CAD build for the part. Positions are in the model's coordinates, mm. Face numbers are marked on the shaded views. A direction names the side the tool comes from. Coordinates: 2 decimals unless noted, no trailing zeros. Order: outer loops, then holes, each group sorted by start corner. A loop starts at its lowest first (then second) coordinate and runs counter-clockwise, first axis right, second up. Notation, with made-up numbers: (-30, 64) - (17, 64) arc R36 cw to (17, 103) - close; hole circle Ø5 at (88, 70.5). An arc over 180 degrees is marked (long way). Use one line per item in the form item = value.
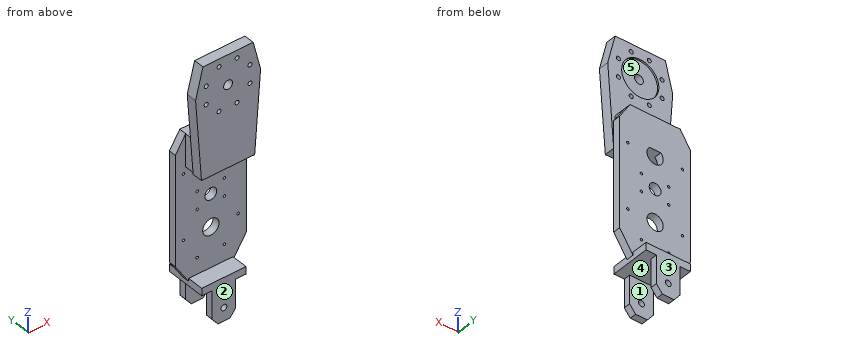
```python
from build123d import *

# Parameters (mm, degrees)
SK_KNEE_PLATE_R         = 2.75
SK_KNEE_PLATE_R_2       = 6
KNEE_PLATE_DEPTH        = 14
SK_KNEE_PILOT_RECESS_R  = 25.15
KNEE_PILOT_RECESS_DEPTH = 2.2
SK_JOGGLE_W             = 68
SK_JOGGLE_H             = 39
JOGGLE_DEPTH            = 44
SK_WEB_R                = 1.7
SK_WEB_R_2              = 11
SK_WEB_R_3              = 8
WEB_DEPTH               = 10
SK_FORK_BAR_W           = 60
SK_FORK_BAR_H           = 54
FORK_BAR_DEPTH          = 10
SK_TINE_LAT_R           = 4
TINE_LAT_DEPTH          = 9
SK_TINE_MED_R           = 4
TINE_MED_DEPTH          = 9


with BuildPart() as part:
    # SK_Knee_Plate → Knee_Plate (new body)
    with BuildSketch(Plane(origin=(0, -34, 0), x_dir=(1, 0, 0), z_dir=(0, 1, 0))):
        Polygon((-34, -40), (34, -40), (44, 0), (36, 110), (-36, 110), (-44, 0), align=None)
        with Locations(Location((29.56414504, 12.245869836, 0), (0, 0, 90))):
            Circle(SK_KNEE_PLATE_R, mode=Mode.SUBTRACT)
        with Locations(Location((12.245869836, 29.56414504, 0), (0, 0, 90))):
            Circle(SK_KNEE_PLATE_R, mode=Mode.SUBTRACT)
        with Locations(Location((-12.245869836, 29.56414504, 0), (0, 0, 90))):
            Circle(SK_KNEE_PLATE_R, mode=Mode.SUBTRACT)
        with Locations(Location((-29.56414504, 12.245869836, 0), (0, 0, 90))):
            Circle(SK_KNEE_PLATE_R, mode=Mode.SUBTRACT)
        with Locations(Location((-29.56414504, -12.245869836, 0), (0, 0, 90))):
            Circle(SK_KNEE_PLATE_R, mode=Mode.SUBTRACT)
        with Locations(Location((-12.245869836, -29.56414504, 0), (0, 0, 90))):
            Circle(SK_KNEE_PLATE_R, mode=Mode.SUBTRACT)
        with Locations(Location((12.245869836, -29.56414504, 0), (0, 0, 90))):
            Circle(SK_KNEE_PLATE_R, mode=Mode.SUBTRACT)
        with Locations(Location((29.56414504, -12.245869836, 0), (0, 0, 90))):
            Circle(SK_KNEE_PLATE_R, mode=Mode.SUBTRACT)
        with Locations(Location((0, 0, 0), (0, 0, 90))):
            Circle(SK_KNEE_PLATE_R_2, mode=Mode.SUBTRACT)
    extrude(amount=KNEE_PLATE_DEPTH)

    # SK_Knee_Pilot_Recess → Knee_Pilot_Recess (cut)
    with BuildSketch(Plane(origin=(0, -20, 0), x_dir=(1, 0, 0), z_dir=(0, 1, 0))):
        with Locations(Location((0, 0, 0), (0, 0, 270))):
            Circle(SK_KNEE_PILOT_RECESS_R)
    extrude(amount=-KNEE_PILOT_RECESS_DEPTH, mode=Mode.SUBTRACT)

    # SK_Joggle → Joggle (add)
    with BuildSketch(Plane.XY.offset(-110)):
        with Locations((0, -14.5)):
            Rectangle(SK_JOGGLE_W, SK_JOGGLE_H)
    extrude(amount=JOGGLE_DEPTH)

    # SK_Web → Web (add)
    with BuildSketch(Plane(origin=(0, -5, 0), x_dir=(1, 0, 0), z_dir=(0, 1, 0))):
        Polygon((-34, 66), (34, 66), (48, 88), (48, 236), (30, 264), (-30, 264), (-48, 236), (-48, 88), align=None)
        with Locations(Location((37, 118, 0), (0, 0, 270))):
            Circle(SK_WEB_R, mode=Mode.SUBTRACT)
        with Locations(Location((18.5, 150.04293994, 0), (0, 0, 270))):
            Circle(SK_WEB_R, mode=Mode.SUBTRACT)
        with Locations(Location((-18.5, 150.04293994, 0), (0, 0, 270))):
            Circle(SK_WEB_R, mode=Mode.SUBTRACT)
        with Locations(Location((-37, 118, 0), (0, 0, 270))):
            Circle(SK_WEB_R, mode=Mode.SUBTRACT)
        with Locations((-18.5, 85.95706006)):
            Circle(SK_WEB_R, mode=Mode.SUBTRACT)
        with Locations((18.5, 85.95706006)):
            Circle(SK_WEB_R, mode=Mode.SUBTRACT)
        with Locations(Location((37, 206, 0), (0, 0, 270))):
            Circle(SK_WEB_R, mode=Mode.SUBTRACT)
        with Locations(Location((18.5, 238.04293994, 0), (0, 0, 270))):
            Circle(SK_WEB_R, mode=Mode.SUBTRACT)
        with Locations(Location((-18.5, 238.04293994, 0), (0, 0, 270))):
            Circle(SK_WEB_R, mode=Mode.SUBTRACT)
        with Locations(Location((-37, 206, 0), (0, 0, 270))):
            Circle(SK_WEB_R, mode=Mode.SUBTRACT)
        with Locations(Location((-18.5, 173.95706006, 0), (0, 0, 270))):
            Circle(SK_WEB_R, mode=Mode.SUBTRACT)
        with Locations(Location((18.5, 173.95706006, 0), (0, 0, 270))):
            Circle(SK_WEB_R, mode=Mode.SUBTRACT)
        with Locations((0, 118)):
            Circle(SK_WEB_R_2, mode=Mode.SUBTRACT)
        with Locations(Location((0, 206, 0), (0, 0, 270))):
            Circle(SK_WEB_R_2, mode=Mode.SUBTRACT)
        with Locations(Location((0, 162, 0), (0, 0, 270))):
            Circle(SK_WEB_R_3, mode=Mode.SUBTRACT)
    extrude(amount=WEB_DEPTH)

    # SK_Fork_Bar → Fork_Bar (add)
    with BuildSketch(Plane.XY.offset(-270)):
        Rectangle(SK_FORK_BAR_W, SK_FORK_BAR_H)
    extrude(amount=FORK_BAR_DEPTH)

    # SK_Tine_Lat → Tine_Lat (add)
    with BuildSketch(Plane(origin=(0, 18, 0), x_dir=(1, 0, 0), z_dir=(0, 1, 0))):
        Polygon((-16, 260), (16, 260), (16, 308), (8, 318), (-8, 318), (-16, 308), align=None)
        with Locations(Location((0, 300, 0), (0, 0, 270))):
            Circle(SK_TINE_LAT_R, mode=Mode.SUBTRACT)
    extrude(amount=TINE_LAT_DEPTH)

    # SK_Tine_Med → Tine_Med (add)
    with BuildSketch(Plane(origin=(0, -27, 0), x_dir=(1, 0, 0), z_dir=(0, 1, 0))):
        Polygon((-16, 260), (16, 260), (16, 308), (8, 318), (-8, 318), (-16, 308), align=None)
        with Locations(Location((0, 300, 0), (0, 0, 270))):
            Circle(SK_TINE_MED_R, mode=Mode.SUBTRACT)
    extrude(amount=TINE_MED_DEPTH)


solid = part.part
```
Item 1: Cut at B-B, the plane z = -291. Write the cut outline in (x, y), plus the area to 3 significant figures.
Derived:
outline = (-16, -27) - (16, -27) - (16, -18) - (-16, -18) - close; (-16, 18) - (16, 18) - (16, 27) - (-16, 27) - close
area = 576 mm²
Item 2: Cut at C-C, the plane y = 22.5. Write the cut outline in (x, z), plus the area to 3 significant figures.
Derived:
outline = (-30, -270) - (-16, -270) - (-16, -308) - (-8, -318) - (8, -318) - (16, -308) - (16, -270) - (30, -270) - (30, -260) - (-30, -260) - close; hole circle Ø8 at (0, -300)
area = 2,010 mm²
Item 3: Two-plate mould, pull along X, no slides. Class the marked faces 4 and 5: +X half, -X half, draft (parallel to the pull), parting line (faces both ways), or undercut.
Derived:
face_4 = draft
face_5 = undercut
Item 4: Cut at D-D, the plane z = -96. Write the cut outline in (x, y).
Derived:
outline = (-48, -5) - (-34, -5) - (-34, -20) - (-37.02, -20) - (-37.02, -34) - (37.02, -34) - (37.02, -20) - (34, -20) - (34, -5) - (48, -5) - (48, 5) - (-48, 5) - close
Item 5: Cut at A-A, the plane y = -9.5. Write the cut outline in (x, z), plus the area to 3 significant figures.
Derived:
outline = (-34, -110) - (34, -110) - (34, -66) - (-34, -66) - close; (-30, -270) - (30, -270) - (30, -260) - (-30, -260) - close
area = 3,590 mm²
Item 6: Drill centre lines: line 1 (Z direction, x = 19, y = -3); line 2 (X direction, y = -0.75, z = -118); line 3 (Z direction, x = -1, y = -18.5). Where is each one in solid material? Low to high. Write a range as [from, to].
Derived:
line_1 = [-270, -239.67], [-236.42, -175.58], [-172.33, -151.67], [-148.42, -66]
line_2 = [-48, -38.7], [-35.3, -11], [11, 35.3], [38.7, 48]
line_3 = [-318, -303.87], [-296.13, -260], [-110, -66]
Item 7: 3-axis set-ups, long thin cutter, end or side, ignore diameter. For the marked faces 1, 2 and 3: which of +Z, -Z, +X, -X, +Y, -Y reach the whole face in a straight line?
Derived:
face_1 = -Z, +X, -X
face_2 = -Z, +X, -X, -Y
face_3 = +Z, -Z, +X, -X, +Y
Item 8: Drop flat-ended pins along their axis: pin 1 (4.5 mm diameter, centred on x = -37, z = -206, fed in from -Y); pin 2 (11 mm diameter, centred on y = 2.5, z = -266.5, fed in from -X); pin 3 (24 mm diameter, centred on x = -4.5, y = -19.5, fed in from +Z); pin 4 (9 mm diameter, centred on x = -29.56, z = -12.25, fed in from +Y). Give the stop position or say it passes through.
Derived:
pin_1 = -5
pin_2 = -31.93
pin_3 = 40
pin_4 = -20
